Build history of the part. All positions in model axes, mm. Face numbers are marked on the shaded views. Give positions to 0.01 mm unless a question says otherwise; leave off trailing zeros. Order: outer loops, then holes, each group sorted by start corner. A loop starts at its lowest first (then second) coordinate and runs counter-clockwise, first axis right, second up. Notation, with made-up numbers: (-25, 89.25) - (-8, 89.25) arc R17 cw to (-8, 117.25) - close; hole circle Ø9 at (76.25, 4.5). An arc over 180 degrees is marked (long way). Use a Markdown table: item, result. Add a question column.
(1) Slice it at A-A (x = 0). Write the cut outline in (y, z).
(2) Mould opens along X. For the marked faces 1, 2 and 3 say: +X half, -X half, draft (parallel to the pull), parting line (faces both ways), or undercut.
(3) Wall check: line 1 (Z direction, x = 28, y = -16); line 2 (X direction, y = 0, z = 2); line 3 (X direction, y = 0, z = 1.4). Give the ranges that are in metal, low to high.
(4) Flat gauge pins, fed straight in: pin 1 (1.5 mm diameter, centred on y = 34.5, z = 63, fed in from -X); pin 2 (12 mm diameter, centred on x = -23, y = 21, fed in from +Z); pin 3 (4 mm diameter, centred on x = -28, y = 22.5, fed in from +Z). Where does each tip first touch, or does it go through?
(5) Slice it at C-C (z = 136). Write the cut outline in (x, y).
(6) Slice it at D-D (z = 47). Write the cut outline in (x, y).
from build123d import *


# Not quite as in the source:
# - a fillet or chamfer that OpenCascade refuses, or shapes differently, is made with other operations: its cross-section is extruded or revolved along the edge and cut away or added


with BuildPart() as f1:
    # F0 (on Front) → F1 (revolve)
    with BuildSketch(Plane.XZ):
        Polygon((-45, 0), (-45, 5), (-44.1333333333, 15), (-32.417820976, 150.1789887381), (-42, 150), (-55, 0), align=None)
        Polygon((-45, 5), (0, 5), (0, 15), (-44.1333333333, 15), align=None)
    revolve(axis=Axis((0, 0, 75), (0, 0, 1)))

    # F2: fillet of radius 20 on 1 edges, made by hand

    # F2_s1 → F2_t2 (revolve, cut)
    with BuildSketch(Plane.XZ):
        with BuildLine():
            ThreePointArc((-33.9760329601, 132.1996196909), (-35.6682042477, 142.1455232835), (-42, 150))
            Line((-42, 150), (-32.417820976, 150.1789887381))
            Line((-32.417820976, 150.1789887381), (-33.9760329601, 132.1996196909))
        make_face()
    revolve(axis=Axis((0, 0, 150.1789887381), (0, 0, 1)), mode=Mode.SUBTRACT)


solid = f1.part
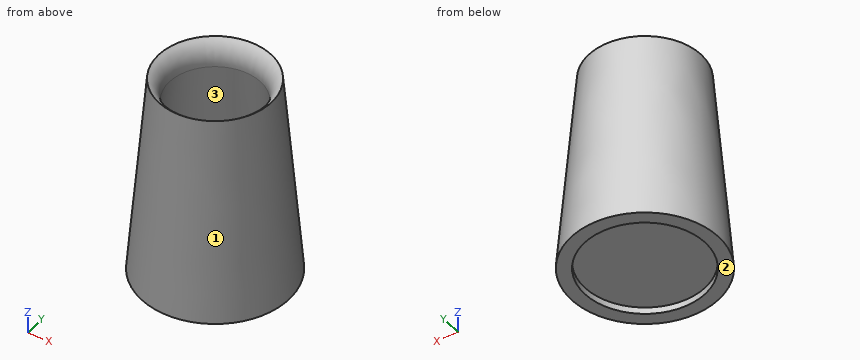
Solution:
| question | item | result |
|---|---|---|
| 1 | outline | (-55, 0) - (-45, 0) - (-45, 5) - (45, 5) - (45, 0) - (55, 0) - (42, 150) arc R20 ccw to (33.98, 132.2) - (44.13, 15) - (-44.13, 15) - (-33.98, 132.2) arc R20 ccw to (-42, 150) - close |
| 2 | face 1 | parting line |
| 2 | face 2 | draft |
| 2 | face 3 | undercut |
| 3 | line 1 | 5 to 15 |
| 3 | line 2 | -54.83 to -45, 45 to 54.83 |
| 3 | line 3 | -54.88 to -45, 45 to 54.88 |
| 4 | pin 1 | x = -36.27 |
| 4 | pin 2 | z = 144.85 |
| 4 | pin 3 | z = 145.95 |
| 5 | outline | circle Ø86.43 at (0, 0); hole circle Ø68.02 at (0, 0) |
| 6 | outline | circle Ø101.85 at (0, 0); hole circle Ø82.72 at (0, 0) |
